Verification items for this drawing (mm, ordinates from the low corner). Give positions to 0.01 mm unless a question says otherwise; leave off trailing zeros. Write each loop counter-clockwise with the first axis right and the second up, starting at its lowest first coordinate (ties: lowest second). Pieces come first, ordered by that corner, then holes. Notation, with made-up numbers: (25, 45.25) -> (53, 45.25) arc R22 cw to (53, 81.25) -> close; hole circle Ø7 at (13.5, 76.25). An arc over 180 degrees is marked (long way). Use one line per item in the form item = value. Start each with the question number.
(1) Depth check by flat-ended pin: pin 1 Ø2.5 at (y, z) = (5, 60) entering from -X. Enter the tip coordinate at first touch or a pass-through.
(2) Section check B-B, the plane x = 0.2. Record the cut outline in (y, z).
(3) Section check C-C, the plane z = 10. Record the cut outline in (x, y).
(4) Scan lines: L1, parallel to Y at x = 0.85, z = 60; L2, parallel to Z at x = 0.95, y = 5.5; L3, parallel to Z at x = 0.8, y = 6. Record each from-to range of solid material in increasing order.
(5) Section check A-A, the plane y = 5. Record the cut outline in (x, z), plus the area to 3 significant figures.
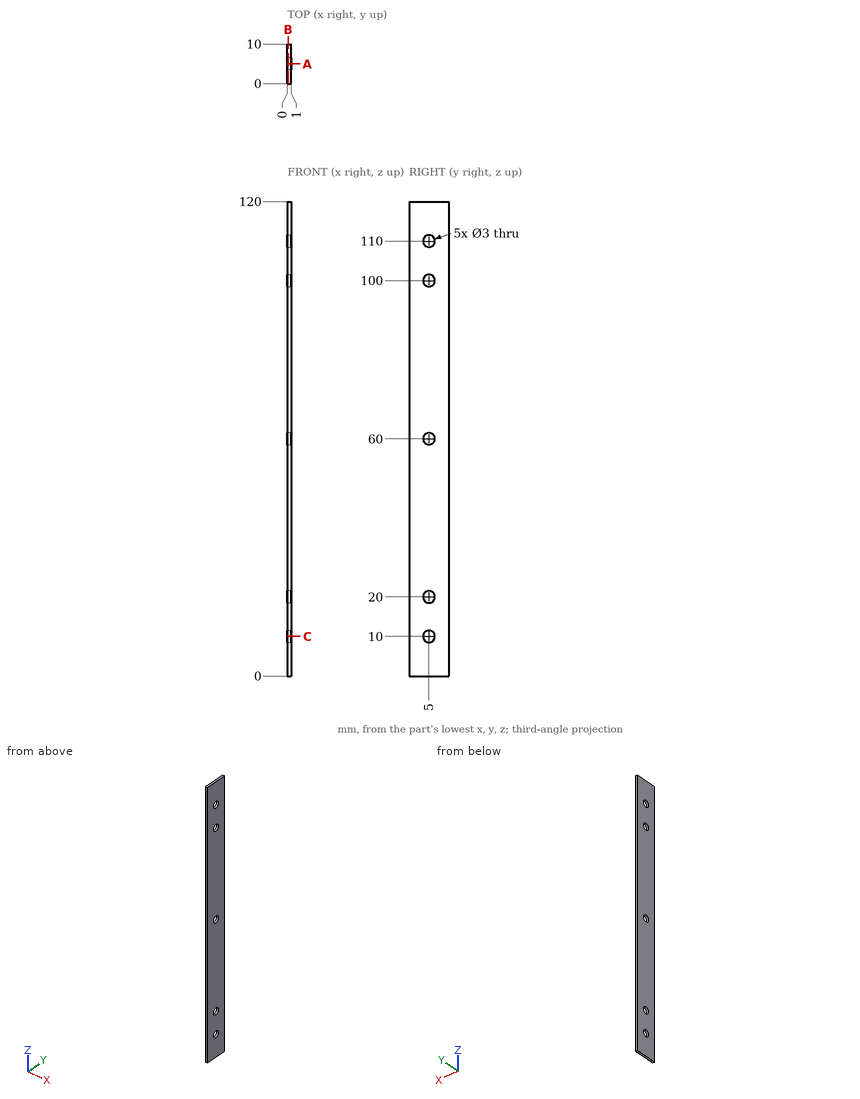
Completed:
q1.pin_1 = through
q2.outline = (0, 0) -> (10, 0) -> (10, 120) -> (0, 120) -> close; hole circle Ø3 at (5, 10); hole circle Ø3 at (5, 20); hole circle Ø3 at (5, 60); hole circle Ø3 at (5, 100); hole circle Ø3 at (5, 110)
q3.outline = (0, 0) -> (1, 0) -> (1, 3.5) -> (0, 3.5) -> close; (0, 6.5) -> (1, 6.5) -> (1, 10) -> (0, 10) -> close
q4.L1 = 0 to 3.5, 6.5 to 10
q4.L2 = 0 to 8.59, 11.41 to 18.59, 21.41 to 58.59, 61.41 to 98.59, 101.41 to 108.59, 111.41 to 120
q4.L3 = 0 to 8.88, 11.12 to 18.88, 21.12 to 58.88, 61.12 to 98.88, 101.12 to 108.88, 111.12 to 120
q5.outline = (0, 0) -> (1, 0) -> (1, 8.5) -> (0, 8.5) -> close; (0, 11.5) -> (1, 11.5) -> (1, 18.5) -> (0, 18.5) -> close; (0, 21.5) -> (1, 21.5) -> (1, 58.5) -> (0, 58.5) -> close; (0, 61.5) -> (1, 61.5) -> (1, 98.5) -> (0, 98.5) -> close; (0, 101.5) -> (1, 101.5) -> (1, 108.5) -> (0, 108.5) -> close; (0, 111.5) -> (1, 111.5) -> (1, 120) -> (0, 120) -> close
q5.area = 105 mm²
